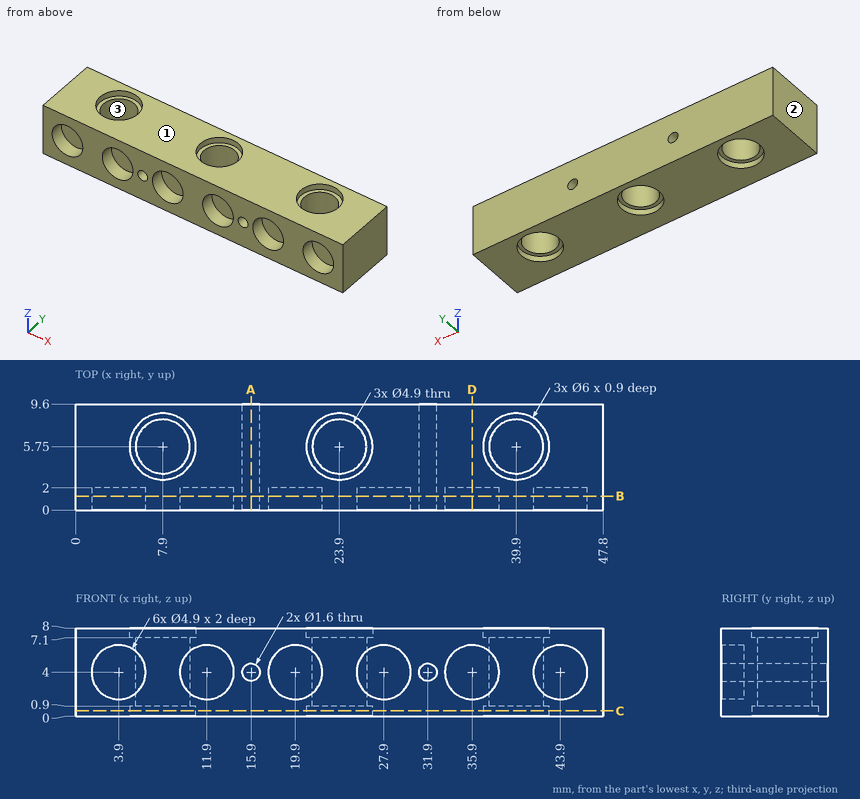
Part print with two shaded views. Sizes in mm from the minimum x, y, z corner. Give positions to 0.01 mm unless a question says otherwise; leave off trailing zeros. Order: outer loops, then holes, each group sorted by start corner. A loop starts at its lowest first (then second) coordinate and runs counter-clockwise, first axis right, second up.
(1) Saw through at B-B, the plane y = 1.25. State how many separate pieces and enclosed holes the cut face has, then the cut area to 3 significant figures.
(2) Drill centre lines: L1, parallel to X at y = 2.25, z = 4; L2, parallel to Z at x = 15.9, y = 4.5; L3, parallel to Y at x = 9, z = 3.75. Where is each one in solid material? Low to high.
(3) Mould opens along X. For the marked faces 1, 2 and 3 say: released by +X, released by -X, zero draft, split by the parting line, or undercut.
(4) Saw through at A-A, the plane x = 15.9. Give the cut face in (y, z).
(5) Flat gauge pins, fed straight in: pin 1 (2.5 mm diameter, centred on x = 20.5, z = 5, fed in from -Y); pin 2 (5 mm diameter, centred on x = 7.9, y = 5.75, fed in from -Z); pin 3 (5.5 mm diameter, centred on x = 7.9, y = 5.75, fed in from +Z). Where does each tip first touch, or does it go through?
(6) Saw through at C-C, the plane z = 0.5. Give the cut face in (x, y).
(7) Saw through at D-D, the plane x = 35.9. Give the cut face in (y, z), then the cut area to 3 significant figures.
Results found:
1. separate pieces: 1
1. enclosed holes: 8
1. area: 265 mm2
2. L1: x = 0 to 15.1, 16.7 to 31.1, 32.7 to 47.8
2. L2: z = 0 to 3.2, 4.8 to 8
2. L3: y = 0 to 3.56, 7.94 to 9.6
3. face 1: zero draft
3. face 2: released by -X
3. face 3: undercut
4. outline: (0, 0) - (9.6, 0) - (9.6, 3.2) - (0, 3.2) - close; (0, 4.8) - (9.6, 4.8) - (9.6, 8) - (0, 8) - close
5. pin 1: stops at y = 2
5. pin 2: stops at z = 0.9
5. pin 3: stops at z = 7.1
6. outline: (0, 0) - (47.8, 0) - (47.8, 9.6) - (0, 9.6) - close; hole circle Ø6 at (7.9, 5.75); hole circle Ø6 at (23.9, 5.75); hole circle Ø6 at (39.9, 5.75)
7. outline: (0, 0) - (9.6, 0) - (9.6, 8) - (0, 8) - (0, 6.45) - (2, 6.45) - (2, 1.55) - (0, 1.55) - close
7. area: 67.0 mm2
